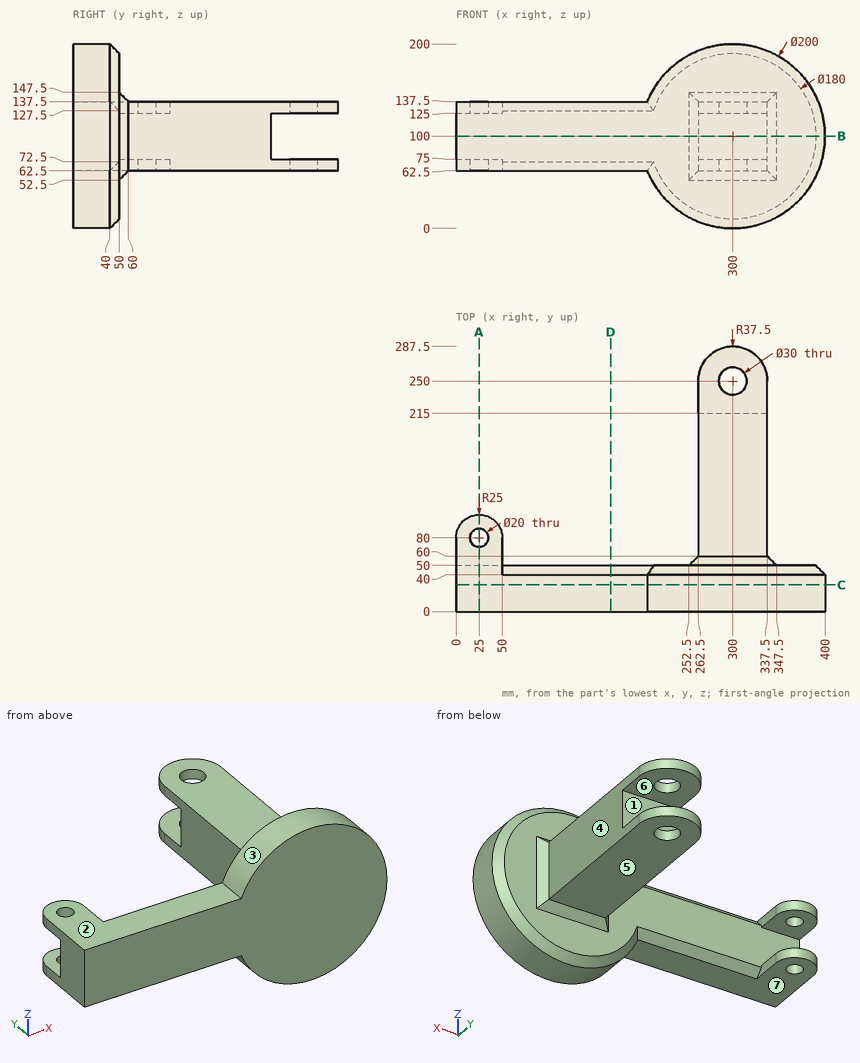
Geometry check sheet. Reference: drawing and pictorial views, mm from the part's lowest x, y, z. A direction names the side the tool comes from. Round coordinates to 2 decimals unless told otherwise and drop trailing zeros. Order: outer loops, then holes, each group sorted by start corner. A loop starts at its lowest first (then second) coordinate and runs counter-clockwise, first axis right, second up.
Q1. Cross-section at A-A, the plane x = 25. Enter the section's corners in (y, z), plus the area to 4 significant figures.
Filled sheet:
outline: (0, 62.5) - (70, 62.5) - (70, 75) - (50, 75) - (50, 125) - (70, 125) - (70, 137.5) - (0, 137.5) - close; (90, 62.5) - (105, 62.5) - (105, 75) - (90, 75) - close; (90, 125) - (105, 125) - (105, 137.5) - (90, 137.5) - close
area: 4,625 mm2
Q2. Scan lines: L1, parallel to X at y = 80, z = 66.5; L2, parallel to Y at x = 300, z = 129; L3, parallel to Y at x = 25, z = 72. Record each from-to range of solid material in increasing order.
Filled sheet:
L1: x = 0 to 15, 35 to 50, 262.5 to 337.5
L2: y = 0 to 235, 265 to 287.5
L3: y = 0 to 70, 90 to 105
Q3. Cross-section at C-C, the plane y = 29. Enter the section's corners in (x, z), plus the area to 3 significant figures.
Filled sheet:
outline: (0, 62.5) - (207.3, 62.5) arc R100 ccw (long way) to (207.3, 137.5) - (0, 137.5) - close
area: 46,600 mm2
Q4. Depth check by flat-ended pin: P1, Ø3, axis at x = 252, z = 154.5, coming from the +Y side; P2, Ø6, axis at x = 339, z = 169, coming from the -Y side; P3, Ø4, axis at y = 63, z = 131, coming from the +X side; P4, Ø15, axis at x = 305, z = 107, coming from the +Y side. Enter the tip coordinate at first touch or a pass-through.
Filled sheet:
P1: stops at y = 50
P2: stops at y = 0
P3: stops at x = 337.5
P4: stops at y = 215
Q5. Set-up check for the marked faces 4, 5, 6 and 7: record each of +Z, -Z, +X, -X, +Y, -Y from which the full face is reachable in a straight line by a thin tool's end or side.
Filled sheet:
face 4: +Z, -Z, +X, +Y
face 5: -Z, +X, -X, +Y
face 6: +X, -X, +Y
face 7: -Z, -X, +Y, -Y
Q6. Draft check along Z on the marked faces 1, 2 and 3. Enter one of: pulls with the +Z half, pulls with the -Z half, needs draft (parallel to the pull), parting line crosses it, or undercut.
Filled sheet:
face 1: undercut
face 2: pulls with the +Z half
face 3: parting line crosses it
Q7. Cross-section at B-B, the plane z = 100. Enter the section's corners in (x, y), plus the area to 3 significant figures.
Filled sheet:
outline: (0, 0) - (400, 0) - (400, 40) - (390, 50) - (347.5, 50) - (337.5, 60) - (337.5, 215) - (262.5, 215) - (262.5, 60) - (252.5, 50) - (0, 50) - close
area: 32,400 mm2
Q8. Cross-section at D-D, the plane x = 167.5. Enter the section's corners in (y, z).
Filled sheet:
outline: (0, 62.5) - (40, 62.5) - (50, 72.5) - (50, 127.5) - (40, 137.5) - (0, 137.5) - close
